```python
from build123d import *

# Parameters (mm, degrees)
MODEL_R             = 1.5
MODEL_R_2           = 1.500000002
MODEL_R_3           = 1.500000008
BOSS_EXTRUDE1_DEPTH = 3


with BuildPart() as part:
    # Model → Boss-Extrude1 (new body)
    with BuildSketch(Plane.XY):
        with BuildLine():
            Line((41.999920867, 34), (41.999920867, 26.34355613))
            ThreePointArc((41.999920867, 26.34355613), (42.930559932, 24.324015901), (44.9959, 23.5))
            Line((44.9959, 23.5), (62.9999, 23.5))
            ThreePointArc((62.9999, 23.5), (65.067553671, 24.322356447), (65.9999, 26.3428))
            Line((65.9999, 26.3428), (65.9999, 34))
            Line((65.9999, 34), (62.9999, 34))
            Line((62.9999, 34), (62.9999, 46))
            Line((62.9999, 46), (65.9999, 46))
            Line((65.9999, 46), (65.9999, 53.6572))
            ThreePointArc((65.9999, 53.6572), (65.068322251, 55.676912854), (63.002020078, 56.5))
            Line((63.002020078, 56.5), (44.993779922, 56.5))
            ThreePointArc((44.993779922, 56.5), (42.930289539, 55.675803247), (41.999920867, 53.65795613))
            Line((41.999920867, 53.65795613), (41.999920867, 46))
            Line((41.999920867, 46), (44.999920867, 46))
            Line((44.999920867, 46), (44.999920867, 34))
            Line((44.999920867, 34), (41.999920867, 34))
        make_face()
        with Locations((45.4999, 53.700050007)):
            Circle(MODEL_R, mode=Mode.SUBTRACT)
        with Locations((62.4999, 53.700099998)):
            Circle(MODEL_R_2, mode=Mode.SUBTRACT)
        with Locations((45.4999, 26.500000005)):
            Circle(MODEL_R_3, mode=Mode.SUBTRACT)
        with Locations((62.4999, 26.500049996)):
            Circle(MODEL_R, mode=Mode.SUBTRACT)
        Polygon((47.8979, 51.3), (47.8979, 28.5), (51.3979, 28.5), (51.3979, 27), (56.3979, 27), (56.3979, 28.5), (60.0979, 28.5), (60.0979, 51.3), align=None, mode=Mode.SUBTRACT)
    extrude(amount=BOSS_EXTRUDE1_DEPTH)


solid = part.part
```
Read the model definition and answer for the solid it produces. Units are mm, in the model's axes. A direction names the side the tool comes from. Give positions to 0.01 mm unless a question says otherwise; leave off trailing zeros. Write each loop counter-clockwise with the first axis right and the second up, starting at its lowest first coordinate (ties: lowest second). Pieces come first, ordered by that corner, then holes. Notation, with made-up numbers: (62.5, 24) -> (86.5, 24) arc R38 cw to (86.5, 63) -> close; hole circle Ø9 at (48.25, -8.5). An arc over 180 degrees is marked (long way). Answer as a JSON object with one key per item and string values.
1) Section C-C on z = 0.75 is taken. Write down the section's boundary in (x, y).
Findings below:
{"outline": "(42, 26.34) arc R3 ccw to (45, 23.5) -> (63, 23.5) arc R3 ccw to (66, 26.34) -> (66, 34) -> (63, 34) -> (63, 46) -> (66, 46) -> (66, 53.66) arc R3 ccw to (63, 56.5) -> (44.99, 56.5) arc R3 ccw to (42, 53.66) -> (42, 46) -> (45, 46) -> (45, 34) -> (42, 34) -> close; hole circle Ø3 at (45.5, 26.5); hole circle Ø3 at (45.5, 53.7); hole (47.9, 28.5) -> (51.4, 28.5) -> (51.4, 27) -> (56.4, 27) -> (56.4, 28.5) -> (60.1, 28.5) -> (60.1, 51.3) -> (47.9, 51.3) -> close; hole circle Ø3 at (62.5, 26.5); hole circle Ø3 at (62.5, 53.7)"}
2) Section A-A on x = 57.5 is taken. Write down the section's boundary in (y, z).
Findings below:
{"outline": "(23.5, 0) -> (28.5, 0) -> (28.5, 3) -> (23.5, 3) -> close; (51.3, 0) -> (56.5, 0) -> (56.5, 3) -> (51.3, 3) -> close"}
3) For a pull along X with two mould halves and no side action, classify faces 6 (the flat face through (58, 28.5, 1)), 7 (the cylindrical face through (44.39, 54.71, 1.48)), 8 (the flat face through (54, 23.5, 1)), 9 (the flat face through (45, 40, 1)) as pulls with the +X half, pulls with the -X half, needs draft (parallel to the pull), parting line crosses it, or undercut.
Findings below:
{"face 6": "undercut", "face 7": "undercut", "face 8": "needs draft", "face 9": "pulls with the -X half"}
4) A tool of negligible diameter and unlimited length cuts with its end or side. For faces 1 (the flat face through (54, 56.5, 1)), 2 (the flat face through (44, 34, 1)), 3 (the flat face through (42, 30, 1)), 4 (the flat face through (60.098, 40, 1)), 5 (the flat face through (65, 34, 1)), from which of +Z, -Z, +X, -X, +Y, -Y can it reach the whole face along a straight path? Write none if from no direction.
Findings below:
{"face 1": "+Z, -Z, +X, -X, +Y", "face 2": "+Z, -Z, -X", "face 3": "+Z, -Z, -X, +Y, -Y", "face 4": "+Z, -Z", "face 5": "+Z, -Z, +X"}
5) Section B-B on y = 36 is taken. Write down the section's boundary in (x, z), then the cut area to 3 significant figures.
Findings below:
{"outline": "(45, 0) -> (47.9, 0) -> (47.9, 3) -> (45, 3) -> close; (60.1, 0) -> (63, 0) -> (63, 3) -> (60.1, 3) -> close", "area": "17.4 mm^2"}
6) Straight lines are drawn through the part: probe 1 along X at (y, z) = (44, 0.8); probe 2 along Y at (x, z) = (48.5, 2.7); probe 3 along X at (y, z) = (52.5, 0.6). For each, find the intervals that lie inside material, in ascending order. Write a range as from..to.
Findings below:
{"probe 1": "x = 45..47.9, 60.1..63", "probe 2": "y = 23.5..28.5, 51.3..56.5", "probe 3": "x = 42..44.6, 46.4..61.6, 63.4..66"}
7) Flat-ended cylindrical pins translate along their axes: pin 1 Ø1.8 at (x, y) = (62.5, 53.7) entering from +Z; pin 2 Ø1.5 at (y, z) = (42, 2) entering from +X; pin 3 Ø3.5 at (x, y) = (45.5, 53.7) entering from -Z; pin 4 Ø1.5 at (x, z) = (44, 1) entering from +Y. Find the tip coordinate at first contact, or state that the pin passes through.
Findings below:
{"pin 1": "passes through", "pin 2": "stops at x = 63", "pin 3": "stops at z = 0", "pin 4": "stops at y = 56.49"}
